Verification items for the finished model (mm, model axes). Face numbers are marked on the shaded views. A direction names the side the tool comes from. Give positions to 0.01 mm unless a question says otherwise; leave off trailing zeros. Loops run counter-clockwise (first coordinate to the right, second up) from the corner with the lowest first, then second, coordinate; pieces in that order, holes last. Notation, with made-up numbers: (26.5, 2.5) - (77.5, 2.5) arc R18 ccw to (77.5, 10.5) - close; hole circle Ø9 at (44.5, 12.25). An arc over 180 degrees is marked (long way). Use one line per item in the form item = value.
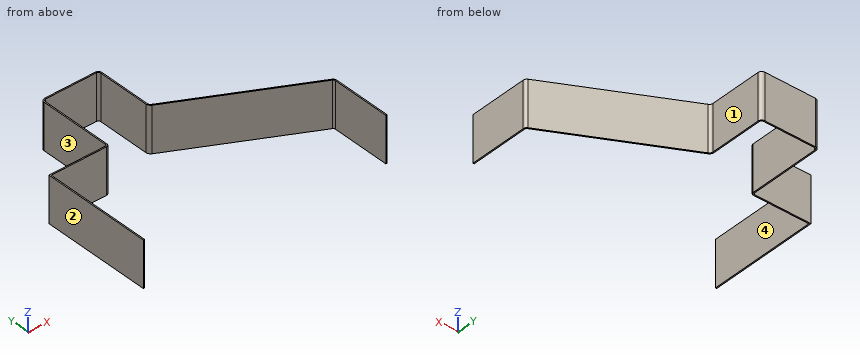
Autodesk Inventor part; units mm, degrees
ref_plane "YZ Plane" through (0, 0, 0) normal (1, 0, 0) x (0, 1, 0)
ref_plane "XZ Plane" through (0, 0, 0) normal (0, 1, 0) x (-1, 0, 0)
ref_plane "XY Plane" through (0, 0, 0) normal (0, 0, 1) x (1, 0, 0)
sketch "Boceto1" plane through (0, 0, 0) normal (0, 0, 1) x (1, 0, 0)
  line L0 (200, -104) -> (200, -8.6304)
  arc A0 (200, -8.6304) -> (196.784, -3.3155) centre (194, -8.6304) ccw
  line L1 (196.784, -3.3155) -> (-6.784, 103.3155)
  arc A1 (-10, 108.6304) -> (-6.784, 103.3155) centre (-4, 108.6304) ccw
  line L2 (-10, 108.6304) -> (-10, 194)
  arc A2 (-10, 194) -> (-16, 200) centre (-16, 194) ccw
  line L3 (-16, 200) -> (-99, 200)
  arc A3 (-99, 200) -> (-105, 194) centre (-99, 194) ccw
  line L4 (-105, 194) -> (-105, 77)
  arc A4 (-107, 75) -> (-105, 77) centre (-107, 77) ccw
  line L5 (-107, 75) -> (-173, 75)
  arc A5 (-175, 123) -> (-177, 125) centre (-177, 123) ccw
  line L6 (-200, 75) -> (-200, -104)
  line L7 (-173, 75) -> (-200, 75)
  line L8 (-198, 73) -> (-173, 73)
  line L9 (-173, 73) -> (-107, 73)
  arc A6 (-107, 73) -> (-103, 77) centre (-107, 77) ccw
  line L10 (-103, 77) -> (-103, 194)
  arc A7 (-99, 198) -> (-103, 194) centre (-99, 194) ccw
  line L11 (-99, 198) -> (-16, 198)
  arc A8 (-12, 194) -> (-16, 198) centre (-16, 194) ccw
  line L12 (-12, 194) -> (-12, 108.6304)
  arc A9 (-12, 108.6304) -> (-7.7121, 101.5438) centre (-4, 108.6304) ccw
  line L13 (-7.7121, 101.5438) -> (195.856, -5.0871)
  arc A10 (198, -8.6304) -> (195.856, -5.0871) centre (194, -8.6304) ccw
  line L14 (198, -8.6304) -> (198, -104)
  line L15 (-198, 73) -> (-198, -104)
  line L16 (-200, -104) -> (-198, -104)
  line L17 (198, -104) -> (200, -104)
  point P0 (0, 0)
  dimension "d3" = 2
  dimension "d4" = 2
extrude "Extrusión1" add sketch "Boceto1" along normal mid plane 75
properties part number "INTERNAL FRAME" material "Acero, carbono"
1. Section check C-C, the plane y = 83.5. Record the cut outline in (x, z).
Result set:
outline = (-105, -37.5) - (-103, -37.5) - (-103, 37.5) - (-105, 37.5) - close; (26.74, -37.5) - (31.05, -37.5) - (31.05, 37.5) - (26.74, 37.5) - close
2. Section check D-D, the plane x = -136. Record the cut outline in (y, z).
Result set:
outline = (73, -37.5) - (75, -37.5) - (75, 37.5) - (73, 37.5) - close
3. Depth check by flat-ended pin: pin 1 Ø1.5 at (x, z) = (134, -5) entering from +Y; pin 2 Ø4 at (y, z) = (122.5, 24) entering from +X; pin 3 Ø3 at (x, z) = (86, -3) entering from +Y. Enter the tip coordinate at first touch or a pass-through.
Result set:
pin_1 = 29.96
pin_2 = -10
pin_3 = 55.5
4. Scan lines: probe 1 along X at (y, z) = (-18, -29); probe 2 along Y at (x, z) = (-177, 34.5); probe 3 along X at (y, z) = (118.5, -21.5). Record each from-to range of solid material in increasing order.
Result set:
probe_1 = -200 to -198, 198 to 200
probe_2 = 73 to 75
probe_3 = -105 to -103, -12 to -10
5. Tool access check on the marked faces 1, 2, 3 and 4. Record the directions out of +Z, -Z, +X, -X, +Y, -Y that give a thin tool (end or side, any length) a straight path to the whole face; none if there is none.
Result set:
face_1 = +Z, -Z, +X, +Y
face_2 = +Z, -Z, -X, +Y, -Y
face_3 = +Z, -Z, -X, +Y
face_4 = +Z, -Z, -Y
6. Section check B-B, the plane z = 29. Record the cut outline in (x, y).
Result set:
outline = (-200, -104) - (-198, -104) - (-198, 73) - (-107, 73) arc R4 ccw to (-103, 77) - (-103, 194) arc R4 cw to (-99, 198) - (-16, 198) arc R4 cw to (-12, 194) - (-12, 108.63) arc R8 ccw to (-7.71, 101.54) - (195.86, -5.09) arc R4 cw to (198, -8.63) - (198, -104) - (200, -104) - (200, -8.63) arc R6 ccw to (196.78, -3.32) - (-6.78, 103.32) arc R6 cw to (-10, 108.63) - (-10, 194) arc R6 ccw to (-16, 200) - (-99, 200) arc R6 ccw to (-105, 194) - (-105, 77) arc R2 cw to (-107, 75) - (-200, 75) - close
7. Section check A-A, the plane y = 155.5. Record the cut outline in (x, z), then the cut area to 3 significant figures.
Result set:
outline = (-105, -37.5) - (-103, -37.5) - (-103, 37.5) - (-105, 37.5) - close; (-12, -37.5) - (-10, -37.5) - (-10, 37.5) - (-12, 37.5) - close
area = 300 mm²
